Build history of the part. All positions in model axes, mm. A direction names the side the tool comes from. Round coordinates to 2 decimals unless told otherwise and drop trailing zeros. Write each loop counter-clockwise with the first axis right and the second up, starting at its lowest first coordinate (ties: lowest second). Pieces come first, ordered by that corner, then holes.
from build123d import *

# Parameters (mm, degrees)
SK_FOREARM_PLATE_W       = 48
SK_FOREARM_PLATE_H       = 208
SK_FOREARM_PLATE_R       = 1.7
SK_FOREARM_PLATE_R_2     = 4
FOREARM_PLATE_DEPTH      = 6
SK_ELBOW_PILOT_RECESS_R  = 12.15
ELBOW_PILOT_RECESS_DEPTH = 2.2
SK_HAND_PLATE_W          = 48
SK_HAND_PLATE_H          = 53.5
SK_HAND_PLATE_R          = 3
HAND_PLATE_DEPTH         = 6


with BuildPart() as part:
    # SK_Forearm_Plate → Forearm_Plate (new body)
    with BuildSketch(Plane(origin=(0, -31.5, 0), x_dir=(1, 0, 0), z_dir=(0, 1, 0))):
        with Locations((0, 76)):
            Rectangle(SK_FOREARM_PLATE_W, SK_FOREARM_PLATE_H)
        with Locations(Location((16, 0, 0), (0, 0, 270))):
            Circle(SK_FOREARM_PLATE_R, mode=Mode.SUBTRACT)
        with Locations(Location((8, 13.856406461, 0), (0, 0, 270))):
            Circle(SK_FOREARM_PLATE_R, mode=Mode.SUBTRACT)
        with Locations(Location((-8, 13.856406461, 0), (0, 0, 270))):
            Circle(SK_FOREARM_PLATE_R, mode=Mode.SUBTRACT)
        with Locations(Location((-16, 0, 0), (0, 0, 270))):
            Circle(SK_FOREARM_PLATE_R, mode=Mode.SUBTRACT)
        with Locations(Location((-8, -13.856406461, 0), (0, 0, 270))):
            Circle(SK_FOREARM_PLATE_R, mode=Mode.SUBTRACT)
        with Locations(Location((8, -13.856406461, 0), (0, 0, 270))):
            Circle(SK_FOREARM_PLATE_R, mode=Mode.SUBTRACT)
        with Locations(Location((0, 0, 0), (0, 0, 270))):
            Circle(SK_FOREARM_PLATE_R_2, mode=Mode.SUBTRACT)
    extrude(amount=FOREARM_PLATE_DEPTH)

    # SK_Elbow_Pilot_Recess → Elbow_Pilot_Recess (cut)
    with BuildSketch(Plane(origin=(0, -25.5, 0), x_dir=(1, 0, 0), z_dir=(0, 1, 0))):
        with Locations(Location((0, 0, 0), (0, 0, 270))):
            Circle(SK_ELBOW_PILOT_RECESS_R)
    extrude(amount=-ELBOW_PILOT_RECESS_DEPTH, mode=Mode.SUBTRACT)

    # SK_Hand_Plate → Hand_Plate (add)
    with BuildSketch(Plane.XY.offset(-186)):
        with Locations((0, -4.75)):
            Rectangle(SK_HAND_PLATE_W, SK_HAND_PLATE_H)
        Circle(SK_HAND_PLATE_R, mode=Mode.SUBTRACT)
    extrude(amount=HAND_PLATE_DEPTH)


solid = part.part
1) Pin check, flat tips, straight feed: pin 1 Ø2 at (x, z) = (-8, -13.86) entering from -Y; pin 2 Ø5.5 at (x, z) = (16, 0) entering from +Y; pin 3 Ø14 at (x, y) = (-3, 8.5) entering from +Z. Stop position of each tip, or through.
Results:
pin 1: passes through
pin 2: stops at y = -25.5
pin 3: stops at z = -180
2) Slice it at D-D (z = -32). Write the cut outline in (x, y), plus the area to 3 significant figures.
Results:
outline: (-24, -31.5) - (24, -31.5) - (24, -25.5) - (-24, -25.5) - close
area: 288 mm2
3) Mould opens along Z. For faces 4 (the cylindrical face through (-8.651, -28.542, 15.427)), 5 (the flat face through (0, 4, -180)), 6 (the flat face through (0, -31.5, -80)) say: released by +Z, released by -Z, zero draft, split by the parting line, or undercut.
Results:
face 4: undercut
face 5: released by +Z
face 6: zero draft
4) Slice it at C-C (y = -18). Write the cut outline in (x, z).
Results:
outline: (-24, -186) - (24, -186) - (24, -180) - (-24, -180) - close
5) Which spindle directions (+Z, -Z, +X, -X, +Y, -Y) get a long thin tool onto all of the face, cutting with end or side? Do faces 1 (the flat face through (0, -25.5, -77)), 2 (the cylindrical face through (-17.66, -28.54, -0.37)), 3 (the cylindrical face through (-4.654, -26.585, 11.224)). Say none if no direction does.
Results:
face 1: +Z, +X, -X, +Y
face 2: +Y, -Y
face 3: +Y
6) Wall check: L1, parallel to X at y = -28.85, z = 0; L2, parallel to Y at x = -9, z = -6.5; L3, parallel to Y at x = 0, z = -181.8. Give the ranges that are in metal, low to high.
Results:
L1: x = -24 to -17.7, -14.3 to -4, 4 to 14.3, 17.7 to 24
L2: y = -31.5 to -27.7
L3: y = -31.5 to -3, 3 to 22
7) Slice it at B-B (x = 0). Write the cut outline in (y, z).
Results:
outline: (-31.5, -186) - (-3, -186) - (-3, -180) - (-25.5, -180) - (-25.5, -12.15) - (-27.7, -12.15) - (-27.7, -4) - (-31.5, -4) - close; (-31.5, 4) - (-27.7, 4) - (-27.7, 12.15) - (-25.5, 12.15) - (-25.5, 28) - (-31.5, 28) - close; (3, -186) - (22, -186) - (22, -180) - (3, -180) - close
8) Slice it at A-A (y = 0). Write the cut outline in (x, z).
Results:
outline: (-24, -186) - (-3, -186) - (-3, -180) - (-24, -180) - close; (3, -186) - (24, -186) - (24, -180) - (3, -180) - close
